Verification items for the finished model (mm, model axes). Round coordinates to 2 decimals unless told otherwise and drop trailing zeros. Order: outer loops, then holes, each group sorted by start corner. A loop starts at its lowest first (then second) coordinate and runs counter-clockwise, first axis right, second up. Notation, with made-up numbers: M 51.5,49 L 66.5,49 A29 ccw 66.5,84 Z; hole C 17,-26.5 d9. An arc over 180 degrees is marked long. Use one line per item in the form item = value. Start each with the question number.
Item 1: Cross-section at A-A on x = 10. Enter the section's corners in (y, z), then the cut area to 3 significant figures.
Item 2: Go/stop test with flat-tipped pins: pin 1 Ø6 at (y, z) = (4, -43.5) entering from +X; pin 2 Ø3 at (x, y) = (9.5, 3) entering from +Z; pin 3 Ø2 at (y, z) = (6, 44.5) entering from +X; pin 4 Ø2 at (x, z) = (11, 26.5) entering from -Y. Record where each tip stops, or that it passes through.
Item 3: Cross-section at B-B on z = 41.5. Enter the section's corners in (x, y).
Item 4: Thickness scan on probe 1 along Z at (x, y) = (10, 1.4); probe 2 along Y at (x, z) = (7, 52); probe 3 along X at (y, z) = (17.25, 10). Record the ranges inside material, lowest first. Write a range as [from, to].
Item 5: Cross-section at C-C on y = 12. Enter the section's corners in (x, z), then the cut area to 3 significant figures.
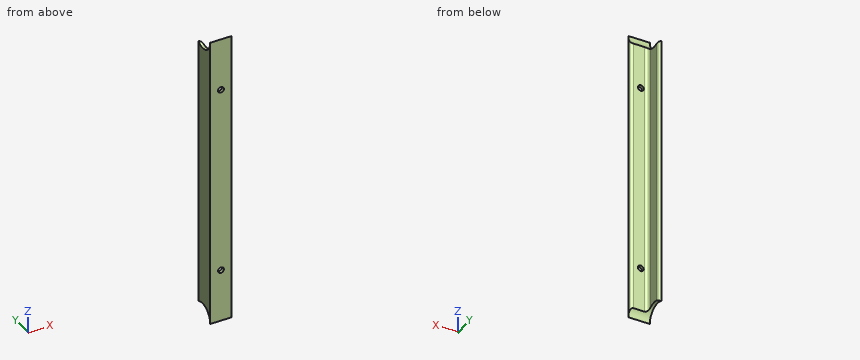
from build123d import *

# Parameters (mm, degrees)
MIEMBRO_ESTRUCTURAL1_DEPTH   = 278.7
CORTAR_EXTRUIR2_DEPTH        = 184.563144285
TALADRO_DE_MARGEN_PARA_M51_D = 5.5


with BuildPart() as part:
    # Sketch1 → Miembro estructural1 (new body)
    with BuildSketch(Plane.XY.offset(-97.329032258)):
        with BuildLine():
            Line((0, 0), (0, 20))
            ThreePointArc((0, 20), (2.121320344, 19.121320344), (3, 17))
            Line((3, 17), (3, 6.5))
            ThreePointArc((3, 6.5), (4.025126266, 4.025126266), (6.5, 3))
            Line((6.5, 3), (17, 3))
            ThreePointArc((17, 3), (19.121320344, 2.121320344), (20, 0))
            Line((20, 0), (0, 0))
        make_face()
    extrude(amount=MIEMBRO_ESTRUCTURAL1_DEPTH)

    # Croquis2 → Cortar-Extruir2 (cut, through all)
    with BuildSketch(Plane.YZ):
        with BuildLine():
            Line((0, -97.329032258), (0, -196.975216041))
            Line((0, -196.975216041), (22.851984592, -196.975216041))
            Line((22.851984592, -196.975216041), (22.851984592, -180.447153459))
            Line((22.851984592, -180.447153459), (12.695152183, -110.128602834))
            ThreePointArc((12.695152183, -110.128602834), (21.887960499, -88.315210983), (0, -97.329032258))
        make_face()
        with BuildLine():
            Line((22.851984592, 264.489088943), (12.695152183, 194.170538318))
            ThreePointArc((12.695152183, 194.170538318), (21.887960499, 172.357146467), (0, 181.370967742))
            Line((0, 181.370967742), (0, 281.017151525))
            Line((0, 281.017151525), (22.851984592, 281.017151525))
            Line((22.851984592, 281.017151525), (22.851984592, 264.489088943))
        make_face()
    extrude(amount=CORTAR_EXTRUIR2_DEPTH, mode=Mode.SUBTRACT)

    # Taladro de margen para M51 (through all)
    with Locations(Plane(origin=(0, 0, 0), x_dir=(-1, 0, 0), z_dir=(0, -1, 0))):
        with Locations((-10, -131.370967742), (-10, 47.329032258)):
            Hole(TALADRO_DE_MARGEN_PARA_M51_D / 2)


solid = part.part
Output values:
q1.outline = M 0,-97.33 A12.8 cw 3,-89.09 L 3,-50.08 L 0,-50.08 Z; M 0,-44.58 L 3,-44.58 L 3,128.62 L 0,128.62 Z; M 0,134.12 L 3,134.12 L 3,173.14 A12.8 cw 0,181.37 Z
q1.area = 769 mm2
q2.pin_1 = 19.83
q2.pin_2 = 175.36
q2.pin_3 = 3.34
q2.pin_4 = 0
q3.outline = M 0,0 L 20,0 A3 ccw 17,3 L 6.5,3 A3.5 cw 3,6.5 L 3,17 A3 ccw 0,20 Z
q4.probe_1 = [-91.51, -50.08], [-44.58, 128.62], [134.12, 175.55]
q4.probe_2 = [0, 3]
q4.probe_3 = [0, 2.99]
q5.outline = M 0,-84.55 L 3,-84.55 L 3,168.6 L 0,168.6 Z
q5.area = 759 mm2
